```python
from build123d import *

# Parameters (mm, degrees)
F1_DEPTH = 228.6
F2_T     = 19.05


with BuildPart() as f1:
    # F0 (on Front) → F1 (new body)
    with BuildSketch(Plane.XZ):
        Polygon((20.4729149157, -8.0454803992), (-3.2688670465, 21.7528046061), (-17.2040478692, -13.7073242069), align=None)
    extrude(amount=F1_DEPTH)

    # F2
    f2_openings = [f1.faces().sort_by_distance(p)[0] for p in [
        (0, 0, 0),
    ]]
    offset(amount=F2_T, openings=f2_openings, kind=Kind.INTERSECTION)


solid = f1.part
```
CAD build for the part. Positions are in the model's coordinates, mm. A direction names the side the tool comes from. Round coordinates to 2 decimals unless told otherwise and drop trailing zeros. Write each loop counter-clockwise with the first axis right and the second up, starting at its lowest first coordinate (ties: lowest second). Pieces come first, ordered by that corner, then holes. Notation, with made-up numbers: M 12.5,4.5 L 31.5,4.5 A7 ccw 31.5,14.5 Z; hole C -20.75,49 d1. An arc over 180 degrees is marked long. One line per question, with ' | ' between items.
1. Cut at A-A on y = -138.5. Write the cut outline in (x, z), and give its area (3 significant figures).
Working result:
outline: M -47,-37.45 L 55.93,-21.98 L -8.93,59.43 Z; hole M -17.2,-13.71 L 20.47,-8.05 L -3.27,21.75 Z | area: 4,060 mm2
2. Cut at B-B on x = 14. Write the cut outline in (y, z).
Working result:
outline: M -247.65,-28.28 L 0,-28.28 L 0,-9.02 L -228.6,-9.02 L -228.6,0.08 L 0,0.08 L 0,30.65 L -247.65,30.65 Z
3. Probe L1, parallel to X at y = -228, z = -5.5; L2, parallel to X at y = -212, z = 14.5; L3, parallel to Z at x = 12, y = -73.5. List the from-to ranges inside material, lowest first. Write a range as from..to.
Working result:
L1: -34.45..-13.98, 18.44..42.8 | L2: -26.59..-6.12, 2.51..26.87 | L3: -28.58..-9.32, 2.59..33.16
4. Cut at C-C on z = 14. Write the cut outline in (x, y).
Working result:
outline: M -26.78,-247.65 L 27.27,-247.65 L 27.27,0 L 2.91,0 L 2.91,-228.6 L -6.32,-228.6 L -6.32,0 L -26.78,0 Z
5. Cut at D-D on z = 51. Write the cut outline in (x, y).
Working result:
outline: M -12.24,-247.65 L -2.21,-247.65 L -2.21,0 L -12.24,0 Z
6. Pin check, flat tips, straight feed: pin 1 Ø3 at (x, z) = (13, 35.5) entering from -Y; pin 2 Ø8 at (x, y) = (-25, -120.5) entering from -Z; pin 3 Ø3 at (x, z) = (-8.5, 1.5) entering from +Y; pin 4 Ø10 at (x, y) = (-7, -159) entering from +Z. Stop position of each tip, or through.
Working result:
pin 1: through | pin 2: z = -34.74 | pin 3: y = -228.6 | pin 4: z = 59.43
7. Which spindle directions (+Z, -Z, +X, -X, +Y, -Y) get a long thin tool onto all of the face, cutting with end or side? Do faces 1 (the flat face through (-27.7, -122.09, 11.67)), 2 (the flat face through (1, -228.6, 0)). Say none if no direction does.
Working result:
face 1: +Z, -X, +Y, -Y | face 2: +Y
8. Mould opens along X. For faces 3 (the flat face through (-8, 0, 12)), 4 (the flat face through (1.371, -112.7, -10.916)), 5 (the flat face through (23.96, -122.09, 18.15)) say: pulls with the +X half, pulls with the -X half, needs draft (parallel to the pull), parting line crosses it, or undercut.
Working result:
face 3: needs draft | face 4: undercut | face 5: pulls with the +X half
